from build123d import *

# Parameters (mm, degrees)
F1_DEPTH = 16
F3_DEPTH = 16
F5_DEPTH = 42
F7_DEPTH = 12


with BuildPart() as f1:
    # F0 (on Top) → F1 (new body)
    with BuildSketch(Plane.XY):
        with BuildLine():
            Line((-48, 32), (-48, -32))
            Line((-48, -32), (48, -32))
            Line((48, -32), (48, -8))
            Line((48, -8), (28, -8))
            ThreePointArc((28, -8), (20, 0), (28, 8))
            Line((28, 8), (48, 8))
            Line((48, 8), (48, 32))
            Line((48, 32), (-48, 32))
        make_face()
    extrude(amount=F1_DEPTH)

    # F2 (on face) → F3 (join)
    with BuildSketch(Plane(origin=(-48, 0, 0), x_dir=(0, -1, 0), z_dir=(-1, 0, 0))):
        Polygon((-32, 64), (-32, 16), (32, 16), (32, 34), (12, 64), align=None)
    extrude(amount=-F3_DEPTH)

    # F4 (on face) → F5 (join)
    with BuildSketch(Plane(origin=(0, 32, 0), x_dir=(-1, 0, 0), z_dir=(0, 1, 0))):
        with BuildLine():
            Line((-8, 16), (32, 16))
            Line((32, 16), (32, 44))
            Line((32, 44), (24, 44))
            ThreePointArc((24, 44), (12, 32), (0, 44))
            Line((0, 44), (-8, 44))
            Line((-8, 44), (-8, 16))
        make_face()
    extrude(amount=-F5_DEPTH)

    # F6 (on face) → F7 (join)
    with BuildSketch(Plane(origin=(0, 32, 0), x_dir=(-1, 0, 0), z_dir=(0, 1, 0))):
        Polygon((-8, 44), (-48, 16), (-8, 16), align=None)
    extrude(amount=-F7_DEPTH)


solid = f1.part
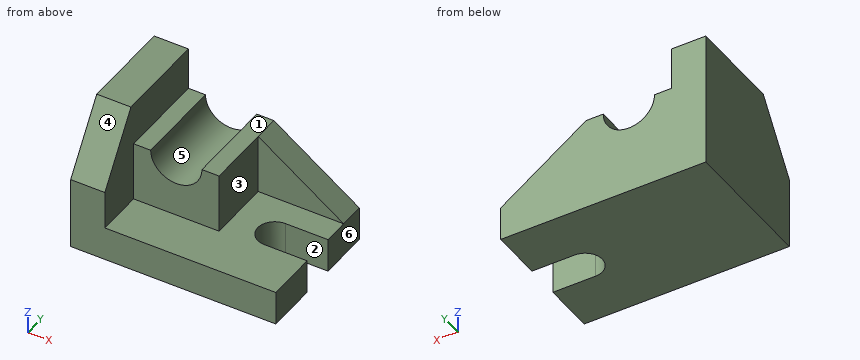
Read the model definition and answer for the solid it produces. Units are mm, in the model's axes. Face numbers are marked on the shaded views. A direction names the side the tool comes from. Round coordinates to 2 decimals unless told otherwise and drop trailing zeros. Write each loop counter-clockwise with the first axis right and the second up, starting at its lowest first coordinate (ties: lowest second). Pieces come first, ordered by that corner, then holes. Notation, with made-up numbers: M 75.25,-20.75 L 99.25,-20.75 A19 cw 99.25,7.25 Z; hole C -21,-20.75 d2. An arc over 180 degrees is marked long. Use a Markdown table: item, result.
1) A tool of negligible diameter and unlimited length cuts with its end or side. For the marked faces 1, 2 and 3, from which of +Z, -Z, +X, -X, +Y, -Y can it reach the whole face along a straight path? Write none if from no direction.
Answers follow:
| item | result |
|---|---|
| face 1 | +Z, +X, +Y, -Y |
| face 2 | +Z, -Z, +X |
| face 3 | +Z, +X, -Y |
2) The part is cut by section A-A (x = 36). Write down the section's boundary in (y, z), plus the area to 3 significant figures.
Answers follow:
| item | result |
|---|---|
| outline | M -32,0 L -8,0 L -8,16 L -32,16 Z; M 8,0 L 32,0 L 32,24.4 L 20,24.4 L 20,16 L 8,16 Z |
| area | 869 mm2 |
3) Flat-ended cylindrical pins translate along their axes: pin 1 (4 mm diameter, centred on y = -7.5, z = 40.5, fed in from +X); pin 2 (8 mm diameter, centred on x = 23, z = 31.5, fed in from -Y); pin 3 (9 mm diameter, centred on x = 5.5, y = 20, fed in from +Z). Find the tip coordinate at first contact, or state that the pin passes through.
Answers follow:
| item | result |
|---|---|
| pin 1 | stops at x = 8 |
| pin 2 | stops at y = 20 |
| pin 3 | stops at z = 44 |
4) Straight lines are drawn through the part: line 1 along X through (y, z) = (-22, 38); line 2 along Z through (x, y) = (-21, -16.5); line 3 along Y through (x, z) = (-9.5, 23). For each, find the intervals that lie inside material, in ascending order. Write a range as [from, to].
Answers follow:
| item | result |
|---|---|
| line 1 | x = [-48, -32] |
| line 2 | z = [0, 16] |
| line 3 | y = [-10, 32] |
5) The part is cut by section C-C (y = 0). Write down the section's boundary in (x, z).
Answers follow:
| item | result |
|---|---|
| outline | M -48,0 L 20,0 L 20,16 L 8,16 L 8,44 L 0,44 A12 cw -24,44 L -32,44 L -32,64 L -48,64 Z |
6) The part is cut by section D-D (z = 14.5). Write down the section's boundary in (x, y).
Answers follow:
| item | result |
|---|---|
| outline | M -48,-32 L 48,-32 L 48,-8 L 28,-8 A8 cw 28,8 L 48,8 L 48,32 L -48,32 Z |
7) The part is cut by section B-B (z = 42.5). Write down the section's boundary in (x, y), plus the area to 3 significant figures.
Answers follow:
| item | result |
|---|---|
| outline | M -48,-26.33 L -32,-26.33 L -32,-10 L -23.91,-10 L -23.91,32 L -48,32 Z; M -0.09,-10 L 8,-10 L 8,20 L 10.14,20 L 10.14,32 L -0.09,32 Z |
| area | 1,640 mm2 |
8) For a pull along X with two mould halves and no side action, classify the marked faces 4, 5 and 6 as pulls with the +X half, pulls with the -X half, needs draft (parallel to the pull), parting line crosses it, or undercut.
Answers follow:
| item | result |
|---|---|
| face 4 | needs draft |
| face 5 | undercut |
| face 6 | pulls with the +X half |
